```python
from build123d import *

# Parameters (mm, degrees)
F0_R     = 70
F0_R_2   = 3
F0_R_3   = 42.5
F1_DEPTH = 3


with BuildPart() as f1:
    # F0 (on Top) → F1 (new body)
    with BuildSketch(Plane.XY):
        Circle(F0_R)
        with Locations((-35.355339, -35.355339)):
            Circle(F0_R_2, mode=Mode.SUBTRACT)
        with Locations((-19.134172, -46.193977)):
            Circle(F0_R_2, mode=Mode.SUBTRACT)
        with Locations((-46.193977, -19.134172)):
            Circle(F0_R_2, mode=Mode.SUBTRACT)
        with Locations((0, -50)):
            Circle(F0_R_2, mode=Mode.SUBTRACT)
        with Locations((19.134172, -46.193977)):
            Circle(F0_R_2, mode=Mode.SUBTRACT)
        with Locations((35.355339, -35.355339)):
            Circle(F0_R_2, mode=Mode.SUBTRACT)
        with Locations((46.193977, -19.134172)):
            Circle(F0_R_2, mode=Mode.SUBTRACT)
        with Locations((-50, 0)):
            Circle(F0_R_2, mode=Mode.SUBTRACT)
        with Locations((-46.193977, 19.134172)):
            Circle(F0_R_2, mode=Mode.SUBTRACT)
        with Locations((-35.355339, 35.355339)):
            Circle(F0_R_2, mode=Mode.SUBTRACT)
        with Locations((-19.134172, 46.193977)):
            Circle(F0_R_2, mode=Mode.SUBTRACT)
        Circle(F0_R_3, mode=Mode.SUBTRACT)
        with Locations((50, 0)):
            Circle(F0_R_2, mode=Mode.SUBTRACT)
        with Locations((46.193977, 19.134172)):
            Circle(F0_R_2, mode=Mode.SUBTRACT)
        with Locations((0, 50)):
            Circle(F0_R_2, mode=Mode.SUBTRACT)
        with Locations((19.134172, 46.193977)):
            Circle(F0_R_2, mode=Mode.SUBTRACT)
        with Locations((35.355339, 35.355339)):
            Circle(F0_R_2, mode=Mode.SUBTRACT)
    extrude(amount=F1_DEPTH)


solid = f1.part
```
Input: part model. Units: mm. Frame: model coordinates. Round coordinates to 2 decimals unless told otherwise and drop trailing zeros. Loops run counter-clockwise (first coordinate to the right, second up) from the corner with the lowest first, then second, coordinate; pieces in that order, holes last. Notation, with made-up numbers: (26.25, 47.25) - (61.25, 47.25) arc R15 cw to (61.25, 76.25) - close; hole circle Ø10 at (77, 61.5). An arc over 180 degrees is marked (long way). One line per item, written item: value. Start each with the question number.
(1) Ray query, line 1 (Y direction, x = 0, z = 2.05); line 2 (Y direction, x = -17, z = 2.5); line 3 (X direction, y = -35, z = 0.15). Return the intervals inside material, ascending. Write a range as [from, to].
(2) Section B-B, the plane z = 2. Count the separate pieces of the cut face and the enclosed holes in it, plus the area to 3 significant figures.
(3) Contact query for flat-ended pins moving along their axis: P1, Ø5.5, axis at x = -35.36, y = 35.36, coming from the -Z side; P2, Ø1.5, axis at x = -22.5, z = 1, coming from the -Y side; P3, Ø1, axis at y = 9.5, z = 2.5, coming from the -X side. Output: stop coordinate, or through.
(4) Draft query along X for faces 1 (the flat face through (-1, -46, 0)), 2 (the cylindrical face through (-21.35, -44.17, 1.48)). Return one class per face: +X half, -X half, draft (parallel to the pull), parting line (faces both ways), or undercut.
(5) Section A-A, the plane y = 0. Return loops of the section in (x, z), plus the area to 3 significant figures.
(6) Section C-C, the plane x = 61.5. Return loops of the section in (y, z), plus the area to 3 significant figures.
Results below:
1. line 1: [-70, -53], [-47, -42.5], [42.5, 47], [53, 70]
1. line 2: [-67.9, -48.3], [-44.09, -38.95], [38.95, 44.09], [48.3, 67.9]
1. line 3: [-60.62, -38.33], [-32.38, -24.11], [24.11, 32.38], [38.33, 60.62]
2. separate pieces: 1
2. enclosed holes: 17
2. area: 9,270 mm^2
3. P1: through
3. P2: y = -66.54
3. P3: x = -69.42
4. face 1: draft
4. face 2: undercut
5. outline: (-70, 0) - (-53, 0) - (-53, 3) - (-70, 3) - close; (-47, 0) - (-42.5, 0) - (-42.5, 3) - (-47, 3) - close; (42.5, 0) - (47, 0) - (47, 3) - (42.5, 3) - close; (53, 0) - (70, 0) - (70, 3) - (53, 3) - close
5. area: 129 mm^2
6. outline: (-33.43, 0) - (33.43, 0) - (33.43, 3) - (-33.43, 3) - close
6. area: 201 mm^2
